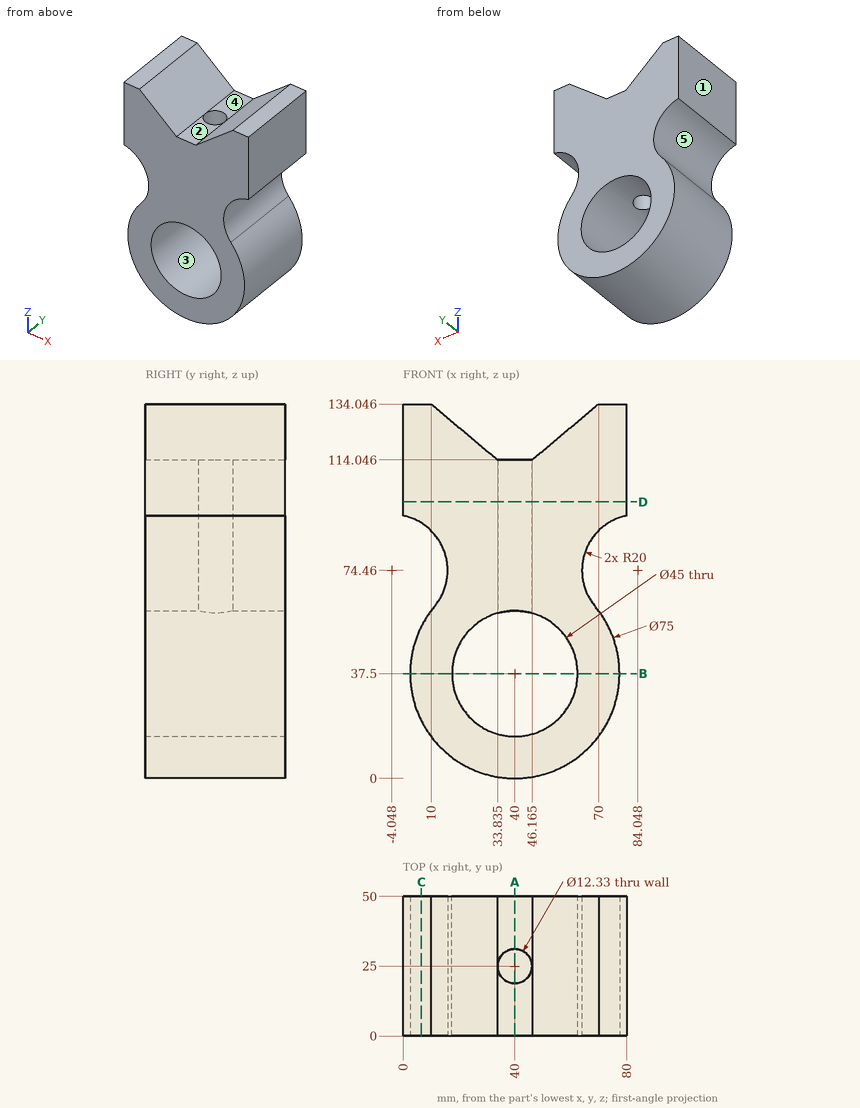
Study the drawing (mm; zero at the part's minimum x, y, z) and answer. A direction names the side the tool comes from. Coordinates: 2 decimals unless noted, no trailing zeros. Write each loop counter-clockwise with the first axis right and the second up, starting at its lowest first coordinate (ties: lowest second). Pieces come first, ordered by that corner, then holes. Notation, with made-up numbers: M 58,39.25 L 102,39.25 A12 ccw 102,49.25 Z; hole C -4.75,78 d8. An arc over 180 degrees is marked long. Write each question's results on one line, items separated by ' | '.
Item 1: For a pull along Z with two mould halves and no side action, classify the marked faces 1, 2 and 3 as released by +Z, released by -Z, zero draft, split by the parting line, or undercut.
Answer below:
face 1: zero draft | face 2: released by +Z | face 3: undercut
Item 2: The part is cut by section B-B on z = 37.5. Determine the outline of the cut face in (x, y), and give its area (3 significant figures).
Answer below:
outline: M 2.5,0 L 17.5,0 L 17.5,50 L 2.5,50 Z; M 62.5,0 L 77.5,0 L 77.5,50 L 62.5,50 Z | area: 1,500 mm2
Item 3: Which of the six approach directions +Z, -Z, +X, -X, +Y, -Y give full straight-line access (tool end or side, diameter ignored) to the marked faces 4 and 5?
Answer below:
face 4: +Z, +Y, -Y | face 5: -X, +Y, -Y
Item 4: The part is cut by section A-A on x = 40. Determine the outline of the cut face in (y, z) (1 decimal), and give its area (3 significant figures).
Answer below:
outline: M 0,0 L 50,0 L 50,15 L 0,15 Z; M 0,60 L 18.8,60 L 18.8,114 L 0,114 Z; M 31.2,60 L 50,60 L 50,114 L 31.2,114 Z | area: 2,790 mm2
Item 5: Given P1, Ø12, axis at y = 24, z = 68, coming from the +X side; P2, Ø3, axis at x = 57, y = 10.5, coming from the +Z side; P3, Ø13.5, axis at x = 42.5, y = 13, coming from the +Z side (1 decimal); P4, Ø2, axis at x = 67, z = 72.5, coming from the +Y side, each flat-ended and moving along its own axis, determine where each tip first touches the part or whether it passes through.
Answer below:
P1: x = 68.4 | P2: z = 124.4 | P3: z = 116.6 | P4: through
Item 6: Consider probe 1 along Y at (x, z) = (40, 90.5) (1 decimal); probe 2 along Z at (x, y) = (40, 15.5); probe 3 along Z at (x, y) = (53.5, 35.5) (1 decimal). Determine where each line is inside the solid, lowest interval first. Write a range as [from, to].
Answer below:
probe 1: [0, 18.8], [31.2, 50] | probe 2: [0, 15], [60, 114.05] | probe 3: [2.5, 19.5], [55.5, 120.2]
Item 7: The part is cut by section D-D on z = 99. Determine the outline of the cut face in (x, y) (1 decimal), and give its area (3 significant figures).
Answer below:
outline: M 0,0 L 80,0 L 80,50 L 0,50 Z; hole C 40,25 d12.3 | area: 3,880 mm2
Item 8: The part is cut by section C-C on x = 6.5. Determine the outline of the cut face in (y, z).
Answer below:
outline: M 0,20.65 L 50,20.65 L 50,54.35 L 0,54.35 Z; M 0,91.45 L 50,91.45 L 50,134.05 L 0,134.05 Z
